Source: CAD feature listing. Evaluate the final solid. Frame: model axes, mm. A direction names the side the tool comes from. Round coordinates to 2 decimals unless told otherwise and drop trailing zeros. Order: outer loops, then holes, each group sorted by start corner. A loop starts at its lowest first (then second) coordinate and runs counter-clockwise, first axis right, second up. Notation, with made-up numbers: (34, -18) - (54, -18) arc R17 cw to (54, -2) - close; hole circle Ø2 at (-29.5, 84.25). An arc over 180 degrees is marked (long way). Return JSON: item names as keys, results as strings. Group by question number.
1) Access query for faces 1 (the flat face through (-0.1, 10.7, 1.5)), 2 (the flat face through (4, 11, 0)), 3 (the cylindrical face through (-5.37, -7.89, 1.19)), 4 (the flat face through (-0.1, 10.7, -1.5)). Directions: +Z, -Z, +X, -X, +Y, -Y. A direction counts if a zero-diameter tool reaches every point of the face in a straight line with its end or side. Return the directions, or none.
2) Ray query, line 1 (Y direction, x = 0, z = -0.35); line 2 (Y direction, x = -2, z = -3); line 3 (Y direction, x = -6.5, z = -1.75). Return the intervals inside material, ascending. Write a range as from..to.
3) Section C-C, the plane x = 6. Return loops of the section in (y, z).
4) Section D-D, the plane y = -5.5. Return loops of the section in (x, z), plus the area to 3 significant figures.
5) Mould query, pull axis Z, two halves, no side actions, for faces 5 (the cylindrical face through (0.33, 3.944, -7.493)), 6 (the flat face through (0, -14, 0)), 7 (the flat face through (-8, 0, 0)), 8 (the cylindrical face through (-1.71, -19.07, 0.38)). Classes: pulls with the +Z half, pulls with the -Z half, needs draft (parallel to the pull), parting line crosses it, or undercut.
6) Section B-B, the plane z = 7. Return loops of the section in (x, y), plus the area to 3 significant figures.
7) Section A-A, the plane y = 13.5. Return loops of the section in (x, z).
8) Contact query for flat-ended pins moving along their axis: P1, Ø6, axis at x = 5, y = -19, coming from the +Z side; P2, Ø8, axis at y = 11.5, z = 3, coming from the -X side; P3, Ø3, axis at x = 0, z = 0, coming from the -Y side. Output: stop coordinate, or through.
```python
from build123d import *

# Parameters (mm, degrees)
ESBO_O1_R                  = 7.5
RESSALTO_EXTRUS_O1_DEPTH   = 8
ESBO_O2_R                  = 8.5
RESSALTO_EXTRUS_O2_DEPTH   = 3
ESBO_O3_W                  = 8
ESBO_O3_H                  = 3
RESSALTO_EXTRUS_O3_DEPTH   = 10
CORTE_EXTRUS_O1_DEPTH      = 23.27666941
CORTE_EXTRUS_O1_DEPTH_BACK = 23.27666941
ESBO_O5_R                  = 3
CORTE_EXTRUS_O2_DEPTH      = 3
ESBO_O6_R                  = 5.5
RESSALTO_EXTRUS_O4_DEPTH   = 10
FILETE1_R                  = 1
SKETCH1_R                  = 1.75
CUT_EXTRUDE1_DEPTH         = 10


with BuildPart() as part:
    # Esboço1 → Ressalto-extrusão1 (new body)
    with BuildSketch(Plane(origin=(0, 0, 0), x_dir=(1, 0, 0), z_dir=(0, 1, 0))):
        with Locations(Location((0, 0, 0), (0, 0, 270))):
            Circle(ESBO_O1_R)
    extrude(amount=RESSALTO_EXTRUS_O1_DEPTH)

    # Esboço2 → Ressalto-extrusão2 (add)
    with BuildSketch(Plane.XZ):
        with Locations(Location((0, 0, 0), (0, 0, 270))):
            Circle(ESBO_O2_R)
    extrude(amount=RESSALTO_EXTRUS_O2_DEPTH)

    # Esboço3 → Ressalto-extrusão3 (add)
    with BuildSketch(Plane(origin=(0, 8, 0), x_dir=(1, 0, 0), z_dir=(0, 1, 0))):
        Rectangle(ESBO_O3_W, ESBO_O3_H)
    extrude(amount=RESSALTO_EXTRUS_O3_DEPTH)

    # Esboço4 → Corte-extrusão1 (cut, two sides: drawn at the far end of the back side and taken through both)
    with BuildSketch(Plane.XY.offset(1.5).offset(-CORTE_EXTRUS_O1_DEPTH_BACK)):
        with BuildLine():
            Line((-4, 18), (-4, 13.999999871))
            ThreePointArc((-4, 13.999999871), (-2.828427176, 16.828427073), (-1.7e-08, 18))
            Line((-1.7e-08, 18), (-4, 18))
        make_face()
        with BuildLine():
            Line((4, 18), (-1.7e-08, 18))
            ThreePointArc((-1.7e-08, 18), (2.828427119, 16.828427131), (4, 14))
            Line((4, 14), (4, 18))
        make_face()
    extrude(amount=CORTE_EXTRUS_O1_DEPTH + CORTE_EXTRUS_O1_DEPTH_BACK, mode=Mode.SUBTRACT)

    # Esboço5 → Corte-extrusão2 (cut)
    with BuildSketch(Plane.XY.offset(1.5)):
        with Locations((0, 14)):
            Circle(ESBO_O5_R)
    extrude(amount=-CORTE_EXTRUS_O2_DEPTH, mode=Mode.SUBTRACT)

    # Esboço6 → Ressalto-extrusão4 (add)
    with BuildSketch(Plane.XZ.offset(3)):
        with Locations(Location((0, 0, 0), (0, 0, 270))):
            Circle(ESBO_O6_R)
    extrude(amount=RESSALTO_EXTRUS_O4_DEPTH)

    # Loft1: read off the stored shape, not the designer's step
    # Loft1: loft between two sections, ruled curve by curve
    loft1_from = [
        Edge.make_bspline([(1.054348973, -13, 5.397994835), (-9.741640698, -13, 7.506692781), (-11.850338644, -13, -3.28929689), (-1.054348973, -13, -5.397994835), (9.741640698, -13, -7.506692781), (11.850338644, -13, 3.28929689), (1.054348973, -13, 5.397994835)], [0, 0, 0, 0, 0.5, 0.5, 0.5, 1, 1, 1, 1], 3, [1, 0.333333333, 0.333333333, 1, 0.333333333, 0.333333333, 1]),
    ]
    loft1_to = [
        Edge.make_bspline([(-0.660465845, -24, 3.945096307), (-8.550658458, -24, 2.624164617), (-7.229726768, -24, -5.266027996), (0.660465845, -24, -3.945096307), (8.550658458, -24, -2.624164617), (7.229726768, -24, 5.266027996), (-0.660465845, -24, 3.945096307)], [0, 0, 0, 0, 0.5, 0.5, 0.5, 1, 1, 1, 1], 3, [1, 0.333333333, 0.333333333, 1, 0.333333333, 0.333333333, 1]),
    ]
    loft1 = Solid(Shell([*[Face.make_surface_from_curves(loft1_from[k], loft1_to[k]) for k in range(1)], Face(Wire(loft1_from)), Face(Wire(loft1_to))]))
    add(loft1)

    # Filete1
    filete1_edges = [part.edges().sort_by_distance(p)[0] for p in [
        (-5.474439314, -13, 0.529635915),
    ]]
    fillet(filete1_edges, radius=FILETE1_R)

    # Sketch1 → Cut-Extrude1 (cut)
    with BuildSketch(Plane.XZ.offset(24)):
        with Locations(Location((0, 0, 0), (0, 0, 270))):
            Circle(SKETCH1_R)
    extrude(amount=-CUT_EXTRUDE1_DEPTH, mode=Mode.SUBTRACT)


solid = part.part
```
Geometry check:
{
 "1": {"face 1": "+Z, +X, -X, +Y", "face 2": "+Z, -Z, +X, +Y", "face 3": "-Y", "face 4": "-Z, +X, -X, +Y"},
 "2": {"line 1": "-14..11, 17..18", "line 2": "-24..8", "line 3": "-3..8"},
 "3": {"outline": "(-3, -6.02) - (0, -6.02) - (0, -4.5) - (8, -4.5) - (8, 4.5) - (0, 4.5) - (0, 6.02) - (-3, 6.02) - close"},
 "4": {"outline": "circle Ø11 at (0, 0)", "area": "95.0 mm2"},
 "5": {"face 5": "parting line crosses it", "face 6": "undercut", "face 7": "needs draft", "face 8": "undercut"},
 "6": {"outline": "(-4.82, -3) - (4.82, -3) - (4.82, 0) - (2.69, 0) - (2.69, 8) - (-2.69, 8) - (-2.69, 0) - (-4.82, 0) - close", "area": "72.0 mm2"},
 "7": {"outline": "(-4, -1.5) - (-2.96, -1.5) - (-2.96, 1.5) - (-4, 1.5) - close; (2.96, -1.5) - (4, -1.5) - (4, 1.5) - (2.96, 1.5) - close"},
 "8": {"P1": "z = 4.22", "P2": "x = -7.42", "P3": "y = -14"}
}
